```python
from build123d import *

# Parameters (mm, degrees)
F0_R      = 12.5
F2_DEPTH  = 2
F3_DEPTH  = 2
F6_DEPTH  = 2
F7_DEPTH  = 2
F9_R      = 3
F8_R      = 1.5
F10_DEPTH = 50
F13_DEPTH = 25
F14_R     = 1.5
F15_DEPTH = 4


with BuildPart() as f2:
    # F0 (on Top) → F2 (new body)
    with BuildSketch(Plane.XY):
        Circle(F0_R)
    extrude(amount=F2_DEPTH)

    # F1 (on Top) → F3 (join)
    with BuildSketch(Plane.XY):
        Polygon((-16, 4.5392797553), (-16, 0), (-16, -5.0607202447), (16, -5.0607202447), (16, 4.5392797553), align=None)
    extrude(amount=F3_DEPTH)

    # F4 (on face) → F6 (join)
    with BuildSketch(Plane.YZ.offset(16)):
        Polygon((-3.447040217, 26), (-5.0607202447, 2), (4.5392797553, 2), (2.552959783, 26), align=None)
    extrude(amount=-F6_DEPTH)

    # F5 (on face) → F7 (join)
    with BuildSketch(Plane(origin=(-16, 0, 0), x_dir=(0, -1, 0), z_dir=(-1, 0, 0))):
        Polygon((-2.552959783, 26), (-4.5392797553, 2), (5.0607202447, 2), (3.447040217, 26), align=None)
    extrude(amount=-F7_DEPTH)

    # F9
    f9_edges = [f2.edges().sort_by_distance(p)[0] for p in [
        (-15, 2.55296, 26),
        (-15, -3.44704, 26),
        (15, 2.55296, 26),
        (15, -3.44704, 26),
    ]]
    fillet(f9_edges, radius=F9_R)

    # F8 (on face) → F10 (cut)
    with BuildSketch(Plane(origin=(-16, 0, 0), x_dir=(0, -1, 0), z_dir=(-1, 0, 0))):
        with Locations((0.447040217, 24)):
            Circle(F8_R)
    extrude(amount=-F10_DEPTH, mode=Mode.SUBTRACT)

    # F12 (on face) → F13 (cut)
    with BuildSketch(Plane(origin=(0, 0, 0), x_dir=(1, 0, 0), z_dir=(0, 0, -1))):
        with BuildLine():
            ThreePointArc((-3.8775368017, 8.6726413711), (-4.6346585758, 6.6910342912), (-2.6530514959, 5.933912517))
            ThreePointArc((-2.6530514959, 5.933912517), (0.2938735431, 6.4933533972), (3.1782167937, 5.670003352))
            ThreePointArc((3.1782167937, 5.670003352), (5.2201137504, 6.2450310193), (4.6450860831, 8.286927976))
            ThreePointArc((4.6450860831, 8.286927976), (0.4295074861, 9.4902857343), (-3.8775368017, 8.6726413711))
        make_face()
        with BuildLine():
            ThreePointArc((-2.6530514959, -5.933912517), (-4.6346585758, -6.6910342912), (-3.8775368017, -8.6726413711))
            ThreePointArc((-3.8775368017, -8.6726413711), (0.4295074861, -9.4902857343), (4.6450860831, -8.286927976))
            ThreePointArc((4.6450860831, -8.286927976), (5.2201137504, -6.2450310193), (3.1782167937, -5.670003352))
            ThreePointArc((3.1782167937, -5.670003352), (0.2938735431, -6.4933533972), (-2.6530514959, -5.933912517))
        make_face()
    extrude(amount=-F13_DEPTH, mode=Mode.SUBTRACT)

    # F14 (on face) → F15 (cut)
    with BuildSketch(Plane(origin=(0, 0, 0), x_dir=(1, 0, 0), z_dir=(0, 0, -1))):
        with BuildLine():
            ThreePointArc((-4.1741742618, -1.4898534581), (-3.0028193225, -1.1205492833), (-2.5, 0))
            ThreePointArc((-2.5, 0), (-3.0028193225, 1.1205492833), (-4.1741742618, 1.4898534581))
            Line((-4.1741742618, 1.4898534581), (-4.1741742618, -1.4898534581))
        make_face()
        with BuildLine():
            Line((-4.1741742618, -1.4898534581), (-4.1741742618, 1.4898534581))
            ThreePointArc((-4.1741742618, 1.4898534581), (-5.5, 0), (-4.1741742618, -1.4898534581))
        make_face()
        with BuildLine():
            ThreePointArc((-4.1741742618, -1.4898534581), (-5.5, 0), (-4.1741742618, 1.4898534581))
            Line((-4.1741742618, 1.4898534581), (-7.8258257382, 1.4898534581))
            ThreePointArc((-7.8258257382, 1.4898534581), (-6.8794507167, 0.9971806775), (-6.5, 0))
            ThreePointArc((-6.5, 0), (-6.8794507167, -0.9971806775), (-7.8258257382, -1.4898534581))
            Line((-7.8258257382, -1.4898534581), (-4.1741742618, -1.4898534581))
        make_face()
        with BuildLine():
            Line((-8.1741742618, 1.4898534581), (-7.8258257382, 1.4898534581))
            ThreePointArc((-7.8258257382, 1.4898534581), (-8, 1.5), (-8.1741742618, 1.4898534581))
        make_face()
        with BuildLine():
            ThreePointArc((-6.5, 0), (-6.8794507167, 0.9971806775), (-7.8258257382, 1.4898534581))
            Line((-7.8258257382, 1.4898534581), (-8.1741742618, 1.4898534581))
            Line((-8.1741742618, 1.4898534581), (-8.1741742618, -1.4898534581))
            Line((-8.1741742618, -1.4898534581), (-7.8258257382, -1.4898534581))
            ThreePointArc((-7.8258257382, -1.4898534581), (-6.8794507167, -0.9971806775), (-6.5, 0))
        make_face()
        with BuildLine():
            ThreePointArc((-8.1741742618, -1.4898534581), (-8, -1.5), (-7.8258257382, -1.4898534581))
            Line((-7.8258257382, -1.4898534581), (-8.1741742618, -1.4898534581))
        make_face()
        with BuildLine():
            Line((-8.1741742618, -1.4898534581), (-8.1741742618, 1.4898534581))
            ThreePointArc((-8.1741742618, 1.4898534581), (-9.5, 0), (-8.1741742618, -1.4898534581))
        make_face()
        with BuildLine():
            ThreePointArc((4.1741742618, 1.4898534581), (4, 1.5), (3.8258257382, 1.4898534581))
            Line((3.8258257382, 1.4898534581), (4.1741742618, 1.4898534581))
        make_face()
        with BuildLine():
            Line((3.8258257382, -1.4898534581), (3.8258257382, 1.4898534581))
            ThreePointArc((3.8258257382, 1.4898534581), (2.5, 0), (3.8258257382, -1.4898534581))
        make_face()
        with BuildLine():
            Line((4.1741742618, 1.4898534581), (3.8258257382, 1.4898534581))
            Line((3.8258257382, 1.4898534581), (3.8258257382, -1.4898534581))
            Line((3.8258257382, -1.4898534581), (4.1741742618, -1.4898534581))
            ThreePointArc((4.1741742618, -1.4898534581), (5.1205492833, -0.9971806775), (5.5, 0))
            ThreePointArc((5.5, 0), (5.1205492833, 0.9971806775), (4.1741742618, 1.4898534581))
        make_face()
        with BuildLine():
            Line((7.8258257382, 1.4898534581), (4.1741742618, 1.4898534581))
            ThreePointArc((4.1741742618, 1.4898534581), (5.1205492833, 0.9971806775), (5.5, 0))
            ThreePointArc((5.5, 0), (5.1205492833, -0.9971806775), (4.1741742618, -1.4898534581))
            Line((4.1741742618, -1.4898534581), (7.8258257382, -1.4898534581))
            ThreePointArc((7.8258257382, -1.4898534581), (6.5, 0), (7.8258257382, 1.4898534581))
        make_face()
        with BuildLine():
            Line((4.1741742618, -1.4898534581), (3.8258257382, -1.4898534581))
            ThreePointArc((3.8258257382, -1.4898534581), (4, -1.5), (4.1741742618, -1.4898534581))
        make_face()
        with BuildLine():
            Line((7.8258257382, -1.4898534581), (7.8258257382, 1.4898534581))
            ThreePointArc((7.8258257382, 1.4898534581), (6.5, 0), (7.8258257382, -1.4898534581))
        make_face()
        with BuildLine():
            ThreePointArc((9.5, 0), (8.9971806775, 1.1205492833), (7.8258257382, 1.4898534581))
            Line((7.8258257382, 1.4898534581), (7.8258257382, -1.4898534581))
            ThreePointArc((7.8258257382, -1.4898534581), (8.9971806775, -1.1205492833), (9.5, 0))
        make_face()
        Circle(F14_R)
    extrude(amount=-F15_DEPTH, mode=Mode.SUBTRACT)


solid = f2.part
```
The listing builds one solid part. Answer for the finished solid, in the listing's coordinates (mm). A direction names the side the tool comes from. Round coordinates to 2 decimals unless told otherwise and drop trailing zeros. Order: outer loops, then holes, each group sorted by start corner. A loop starts at its lowest first (then second) coordinate and runs counter-clockwise, first axis right, second up. Notation, with made-up numbers: (-20, 86.25) - (-11, 86.25) arc R25 ccw to (-11, 121.25) - close; hole circle Ø11 at (-32, 26). An arc over 180 degrees is marked (long way). Put each result on its own line as item: value. Start each with the question number.
(1) Find section A-A (x = 0). Give the vertices of the cut face in (y, z).
(2) Find section D-D (x = 14.5). Give the vertices of the cut face in (y, z), plus the area to 3 significant figures.
(3) Given P1, Ø2, axis at x = 5, z = 1.5, coming from the +Y side; P2, Ø1.6, axis at x = 13.5, z = 1.5, coming from the +Y side; P3, Ø8, axis at x = 8.5, z = 3, coming from the +Y side; P4, Ø3.5, axis at y = -0.45, z = 24, coming from the -X side, each flat-ended and moving along its own axis, determine where each tip first touches the part or whether it passes through.
(4) For faces 1 (the flat face through (-6, 1.49, 1)), 2 (the flat face through (15.014, 3.672, 12.475)), 3 (the flat face through (-14, 4.539, 1)), 4 (the flat face through (0, -3, 2)), 5 (the flat face through (-14, -5.061, 1)), determine the directions among +Z, -Z, +X, -X, +Y, -Y from which every point of the face is accessible in a straight line to the end or side of a thin tool.
(5) Find section B-B (z = 19.5). Give the vertices of the cut face in (x, y), plus the area to 3 significant figures.
(6) Determine the mould class of faces 6 (the cylindrical face through (0.252, -6.495, 0.986)), 7 (the flat face through (-15.01, -4.36, 12.45)), 8 (the flat face through (-16, 0, 10)) for opening direction X: released by +X, released by -X, zero draft, split by the parting line, or undercut.
(7) Find section C-C (y = -7.5). Give the vertices of the cut face in (x, z), plus the area to 3 significant figures.
(8) Straight lines are drawn through the part: probe 1 along Y at (x, z) = (0, 1.2); probe 2 along X at (y, z) = (0.5, 6.25); probe 3 along Z at (x, y) = (3.5, -9.25). For each, find the intervals that lie inside material, in ascending order. Write a range as from..to.
Reply:
1. outline: (-12.5, 0) - (-9.5, 0) - (-9.5, 2) - (-12.5, 2) - close; (-6.5, 0) - (-1.5, 0) - (-1.5, 2) - (-6.5, 2) - close; (1.5, 0) - (6.5, 0) - (6.5, 2) - (1.5, 2) - close; (9.5, 0) - (12.5, 0) - (12.5, 2) - (9.5, 2) - close
2. outline: (-5.06, 0) - (4.54, 0) - (4.54, 2) - (2.78, 23.25) arc R3 ccw to (-0.21, 26) - (-0.64, 26) arc R3 ccw to (-3.64, 23.2) - (-5.06, 2) - close; hole circle Ø3 at (-0.45, 24)
2. area: 196 mm^2
3. P1: y = 11.84
3. P2: y = 4.54
3. P3: y = 11.61
3. P4: x = -16
4. face 1: +Z, -Z
4. face 2: +Z, +X, -X, +Y
4. face 3: +Z, -Z, -X, +Y
4. face 4: +Z, +Y, -Y
4. face 5: +Z, -Z, -X, -Y
5. outline: (-16, -3.88) - (-14, -3.88) - (-14, 3.09) - (-16, 3.09) - close; (14, -3.88) - (16, -3.88) - (16, 3.09) - (14, 3.09) - close
5. area: 27.9 mm^2
6. face 6: undercut
6. face 7: zero draft
6. face 8: released by -X
7. outline: (-10, 0) - (-4.75, 0) - (-4.75, 2) - (-10, 2) - close; (5.32, 0) - (10, 0) - (10, 2) - (5.32, 2) - close
7. area: 19.9 mm^2
8. probe 1: -12.5..-9.5, -6.5..-1.5, 1.5..6.5, 9.5..12.5
8. probe 2: -16..-14, 14..16
8. probe 3: 0..2
